from build123d import *

# Parameters (mm, degrees)
CUT_EXTRUDE6_DEPTH      = 22.692020107
CUT_EXTRUDE6_DEPTH_BACK = 22.692020107


with BuildPart() as part:
    # Sketch11 → Revolve3 (revolve)
    with BuildSketch(Plane(origin=(0, 0, 0), x_dir=(1, 0, 0), z_dir=(0, 1, 0)), mode=Mode.PRIVATE) as revolve3_sk:
        Polygon((14.2748, -7.9375), (14.2748, -2.4010112), (14.2748, 0), (12.7, 0), (12.7, -0.381), (9.652, -0.381), (9.652, 0), (0, 0), (0, -7.9375), (9.652, -7.9375), (9.652, -7.5565), (12.7, -7.5565), (12.7, -7.9375), align=None)
    revolve(revolve3_sk.sketch.rotate(Axis((0, 0, 0.717728402), (0, 0, 1)), 180), axis=Axis((0, 0, 0.717728402), (0, 0, 1)))

    # Sketch12 → Cut-Extrude6 (cut, two sides: drawn at the far end of the back side and taken through both)
    with BuildSketch(Plane(origin=(0, 0, 0), x_dir=(-1, 0, 0), z_dir=(0, 0, 1)).offset(-CUT_EXTRUDE6_DEPTH_BACK)):
        Polygon((7.332348419, 0), (3.666174209, 6.35), (-3.666174209, 6.35), (-7.332348419, 0), (-3.666174209, -6.35), (3.666174209, -6.35), align=None)
    extrude(amount=CUT_EXTRUDE6_DEPTH + CUT_EXTRUDE6_DEPTH_BACK, mode=Mode.SUBTRACT)


solid = part.part
Can you work these out from the model? Positions are in its coordinate system, mm. A direction names the side the tool comes from. Give positions to 0.01 mm unless a question says otherwise; leave off trailing zeros. Write each loop counter-clockwise with the first axis right and the second up, starting at its lowest first coordinate (ties: lowest second). Pieces come first, ordered by that corner, then holes. Notation, with made-up numbers: M 69,33.5 L 106,33.5 A33 ccw 106,72.5 Z; hole C 47.5,-15.75 d3. An arc over 180 degrees is marked long. Answer in a Markdown table with one row per item. Add a question column.
Item 1: For pin 1 Ø2 at (y, z) = (10.5, 5) entering from +X; pin 2 Ø2 at (y, z) = (-4.5, 3.5) entering from -X; pin 3 Ø1 at (y, z) = (-8, 7) entering from +X, each with a flat end and sliding along its axis, tell me the tip position at first contact or that it passes through.
Item 2: Imagine slicing it at A-A, the plane x = 0. Write out the boundary of the cut face in (y, z).
Item 3: Imagine slicing it at C-C, the plane y = -5.5. Write out the boundary of the cut face in (x, z), plus the area to 3 significant figures.
Item 4: We'd pull the mould along Y, two halves only. Please class faces 1 (the flat face through (5.474, -3.219, 3.913)), 2 (the flat face through (-13, 1, 7.938)), 3 (the cylindrical face through (14.26, -0.63, 3.91)), 4 (the cylindrical face through (-5.86, 11.267, 7.75)): released by +Y, released by -Y, zero draft, split by the parting line, or undercut.
Item 5: Please list where these lines run through material, in increasing order: L1, parallel to Y at x = 0, z = 7.7; L2, parallel to X at y = 7.75, z = 7.75; L3, parallel to X at y = -3.5, z = 1.5.
Item 6: Imagine slicing it at D-D, the plane y = 11.25. Write out the boundary of the cut face in (x, z), plus the area to 3 significant figures.
Item 7: Imagine slicing it at B-B, the plane z = 6.75. Write out the boundary of the cut face in (x, y), plus the area to 3 significant figures.
Item 8: On a 3-axis mill with a long thin cutter (end or side, diameter ignored), from which of +Z, -Z, +X, -X, +Y, -Y can I reach the whole of each face in a straight line? I mean faces 5 (the flat face through (-2.8, -9.5, 0.381)), 6 (the flat face through (5.525, 3.131, 3.913)), 7 (the cylindrical face through (7.66, 5.87, 7.74)), 8 (the flat face through (6.3, -2.3, 7.938)). Say none if no direction works.
Evaluation:
| question | item | result |
|---|---|---|
| 1 | pin 1 | stops at x = 10.65 |
| 1 | pin 2 | stops at x = -13.84 |
| 1 | pin 3 | stops at x = 12.15 |
| 2 | outline | M -14.27,0 L -12.7,0 L -12.7,0.38 L -9.65,0.38 L -9.65,0 L -6.35,0 L -6.35,7.94 L -9.65,7.94 L -9.65,7.56 L -12.7,7.56 L -12.7,7.94 L -14.27,7.94 Z; M 6.35,0 L 9.65,0 L 9.65,0.38 L 12.7,0.38 L 12.7,0 L 14.27,0 L 14.27,7.94 L 12.7,7.94 L 12.7,7.56 L 9.65,7.56 L 9.65,7.94 L 6.35,7.94 Z |
| 3 | outline | M -13.17,0 L -11.45,0 L -11.45,0.38 L -7.93,0.38 L -7.93,0 L -4.16,0 L -4.16,7.94 L -7.93,7.94 L -7.93,7.56 L -11.45,7.56 L -11.45,7.94 L -13.17,7.94 Z; M 4.16,0 L 7.93,0 L 7.93,0.38 L 11.45,0.38 L 11.45,0 L 13.17,0 L 13.17,7.94 L 11.45,7.94 L 11.45,7.56 L 7.93,7.56 L 7.93,7.94 L 4.16,7.94 Z |
| 3 | area | 138 mm² |
| 4 | face 1 | undercut |
| 4 | face 2 | zero draft |
| 4 | face 3 | split by the parting line |
| 4 | face 4 | undercut |
| 5 | L1 | y = -14.27 to -12.7, -9.65 to -6.35, 6.35 to 9.65, 12.7 to 14.27 |
| 5 | L2 | x = -11.99 to -10.06, -5.75 to 5.75, 10.06 to 11.99 |
| 5 | L3 | x = -13.84 to -5.31, 5.31 to 13.84 |
| 6 | outline | M -8.79,0 L -5.89,0 L -5.89,0.38 L 5.89,0.38 L 5.89,0 L 8.79,0 L 8.79,7.94 L 5.89,7.94 L 5.89,7.56 L -5.89,7.56 L -5.89,7.94 L -8.79,7.94 Z |
| 6 | area | 131 mm² |
| 7 | outline | C 0,0 d28.55; hole M -7.33,0 L -3.67,-6.35 L 3.67,-6.35 L 7.33,0 L 3.67,6.35 L -3.67,6.35 Z |
| 7 | area | 500 mm² |
| 8 | face 5 | -Z |
| 8 | face 6 | +Z, -Z |
| 8 | face 7 | +Z |
| 8 | face 8 | +Z, +X, -X, +Y, -Y |
